from build123d import *

# Parameters (mm, degrees)
BOSS_EXTRUDE1_DEPTH = 5
FILLET8_R           = 2.5
SKETCH5_R           = 1.25
CUT_EXTRUDE4_DEPTH  = 24.289688565
SKETCH6_R           = 1.25
CUT_EXTRUDE5_DEPTH  = 24.523330833
FILLET9_R           = 0.75
FILLET10_R          = 0.5
SKETCH7_R           = 1.25
CUT_EXTRUDE6_DEPTH  = 1
FILLET11_R          = 0.75
FILLET12_R          = 0.25


with BuildPart() as part:
    # Sketch1 → Boss-Extrude1 (new body)
    with BuildSketch(Plane.XY):
        Polygon((-15.064601776, 1.25), (-15.064601776, -1.25), (14.935398224, -1.25), (14.935398224, -2.5), (22.435398224, -2.5), (22.435398224, -1.25), (16.185398224, -1.25), (16.185398224, 0), (16.185398224, 1.25), (22.435398224, 1.25), (22.435398224, 2.5), (14.935398224, 2.5), (14.935398224, 1.25), align=None)
    extrude(amount=BOSS_EXTRUDE1_DEPTH)

    # Fillet8
    fillet8_edges = [part.edges().sort_by_distance(p)[0] for p in [
        (22.435398224, -1.875, 5),
        (22.435398224, -1.875, 0),
        (22.435398224, 1.875, 0),
        (22.435398224, 1.875, 5),
        (-15.064601776, 0, 0),
        (-15.064601776, 0, 5),
    ]]
    fillet(fillet8_edges, radius=FILLET8_R - 0.0001)  # a hair under: the kernel refuses the full size

    # Sketch5 → Cut-Extrude4 (cut, through all)
    with BuildSketch(Plane(origin=(0, 1.25, 0), x_dir=(1, 0, 0), z_dir=(0, 1, 0))):
        with Locations(Location((-12.564601776, -2.5, 0), (0, 0, 270))):
            Circle(SKETCH5_R)
    extrude(amount=-CUT_EXTRUDE4_DEPTH, mode=Mode.SUBTRACT)

    # Sketch6 → Cut-Extrude5 (cut, through all)
    with BuildSketch(Plane(origin=(0, 2.5, 0), x_dir=(1, 0, 0), z_dir=(0, 1, 0))):
        with Locations(Location((19.935398224, -2.5, 0), (0, 0, 270))):
            Circle(SKETCH6_R)
    extrude(amount=-CUT_EXTRUDE5_DEPTH, mode=Mode.SUBTRACT)

    # Fillet9
    fillet9_edges = [part.edges().sort_by_distance(p)[0] for p in [
        (14.935398224, 2.5, 2.5),
        (14.935398224, -2.5, 2.5),
    ]]
    fillet(fillet9_edges, radius=FILLET9_R)

    # Fillet10
    fillet10_edges = [part.edges().sort_by_distance(p)[0] for p in [
        (14.935398224, -1.25, 2.5),
        (14.935398224, 1.25, 2.5),
    ]]
    fillet(fillet10_edges, radius=FILLET10_R - 0.0001)  # a hair under: the kernel refuses the full size

    # Sketch7 → Cut-Extrude6 (cut)
    with BuildSketch(Plane(origin=(0, 1.25, 0), x_dir=(1, 0, 0), z_dir=(0, 1, 0))):
        with Locations(Location((-12.564601776, -2.5, 0), (0, 0, 270))):
            Circle(SKETCH7_R)
        with BuildLine():
            Line((-8.564601776, -1), (12.435398224, -1))
            ThreePointArc((12.435398224, -1), (13.935398224, -2.5), (12.435398224, -4))
            Line((12.435398224, -4), (-8.564601776, -4))
            ThreePointArc((-8.564601776, -4), (-10.064601776, -2.5), (-8.564601776, -1))
        make_face()
    cut_extrude6 = extrude(amount=-CUT_EXTRUDE6_DEPTH, mode=Mode.SUBTRACT)

    # Mirror2: Cut-Extrude6 across plane
    add(cut_extrude6.mirror(Plane.ZX), mode=Mode.SUBTRACT)

    # Fillet11
    fillet11_edges = [part.edges().sort_by_distance(p)[0] for p in [
        (-10.064601776, 0.25, 2.5),
        (1.935398224, 0.25, 1),
        (13.935398224, 0.25, 2.5),
        (1.935398224, 0.25, 4),
        (-10.064601776, -0.25, 2.5),
        (1.935398224, -0.25, 4),
        (13.935398224, -0.25, 2.5),
        (1.935398224, -0.25, 1),
    ]]
    fillet(fillet11_edges, radius=FILLET11_R)

    # Fillet12
    fillet12_edges = [part.edges().sort_by_distance(p)[0] for p in [
        (1.935398224, -1.25, 1),
        (13.935398224, -1.25, 2.5),
        (1.935398224, -1.25, 4),
        (1.935398224, 1.25, 1),
        (13.935398224, 1.25, 2.5),
        (1.935398224, 1.25, 4),
        (-10.064601776, -1.25, 2.5),
        (-10.064601776, 1.25, 2.5),
    ]]
    fillet(fillet12_edges, radius=FILLET12_R - 0.0001)  # a hair under: the kernel refuses the full size


solid = part.part
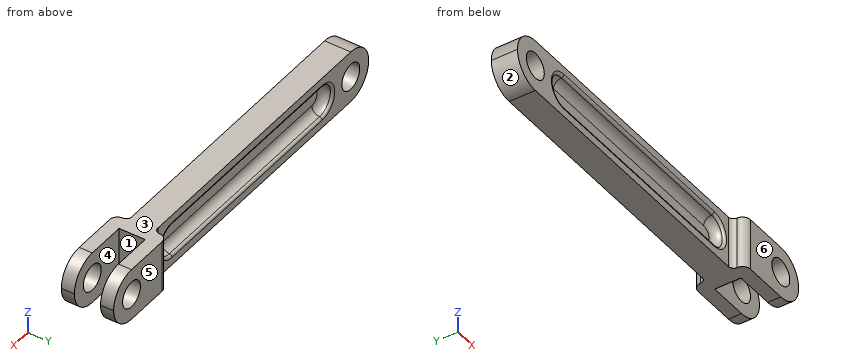
Model file for the job. Use its own axes, mm. Face numbers are marked on the shaded views. A direction names the side the tool comes from. Coordinates: 2 decimals unless noted, no trailing zeros. One line per item, written item: value. Start each with the question number.
1) Probe probe 1 along Z at (x, y) = (20, 1.8); probe 2 along Y at (x, z) = (16.5, 4.3); probe 3 along X at (y, z) = (-0.35, 2.5). List the from-to ranges inside material, lowest first.
2) Slice it at C-C on y = 0.6. Count the separate pieces of the cut face and the enclosed holes in it, then the cut area to 3 significant figures.
3) Flat gauge pins, fed straight in: pin 1 Ø0.8 at (y, z) = (0.5, 2.5) entering from +X; pin 2 Ø2 at (x, z) = (19.94, 2.5) entering from -Y; pin 3 Ø0.8 at (x, z) = (3, 3) entering from -Y; pin 4 Ø1 at (x, z) = (-11, 0.5) entering from +Y. Where does each tip first touch, or does it go through?
4) Pull direction Y, two halves, no side cores. Call the marked faces 3, 4, 5 and 6: +Y half, -Y half, draft (parallel to the pull), parting line (faces both ways), or undercut.
5) Which spindle directions (+Z, -Z, +X, -X, +Y, -Y) get a long thin tool onto all of the face, cutting with end or side? Do the marked faces 1 and 2. Say none if no direction does.
Answers follow:
1. probe 1: 0 to 1.25, 3.75 to 5
1. probe 2: -2.5 to -1.25, 1.25 to 2.5
1. probe 3: -15.06 to -13.81, -11.31 to -9.69, 13.56 to 16.19
2. separate pieces: 1
2. enclosed holes: 2
2. area: 84.5 mm2
3. pin 1: x = 16.19
3. pin 2: through
3. pin 3: y = -0.27
3. pin 4: y = 1.25
4. face 3: draft
4. face 4: undercut
4. face 5: +Y half
4. face 6: -Y half
5. face 1: +Z, -Z, +X
5. face 2: -Z, -X, +Y, -Y
